The listing builds one solid part. Answer for the finished solid, in the listing's coordinates (mm). A direction names the side the tool comes from. Coordinates: 2 decimals unless noted, no trailing zeros. Loops run counter-clockwise (first coordinate to the right, second up) from the corner with the lowest first, then second, coordinate; pieces in that order, holes last. Notation, with made-up numbers: (82.25, 45.25) - (103.25, 45.25) arc R26 ccw to (103.25, 80.25) - close; hole circle Ø5 at (-13, 5). An arc over 180 degrees is marked (long way). Write each question's results on one line, items separated by ' | '. Start each with the question number.
(1) Given pin 1 Ø2.5 at (x, y) = (0, -5) entering from +Z; pin 2 Ø3 at (x, z) = (0.5, 10) entering from +Y; pin 3 Ø4.5 at (x, y) = (0, 9) entering from -Z, each flat-ended and moving along its own axis, determine where each tip first touches the part or whether it passes through.
(2) Find section D-D on y = -9. Determine the outline of the cut face in (x, z), then the cut area to 3 significant figures.
(3) For faces 4 (the cylindrical face through (-0.07, -3.38, 66.9)), 5 (the flat face through (-0.1, 6.8, 17)), 6 (the flat face through (0, 4, 65)), determine the directions among +Z, -Z, +X, -X, +Y, -Y from which every point of the face is accessible in a straight line to the end or side of a thin tool.
(4) Find section B-B on y = 5.25. Determine the outline of the cut face in (x, z).
(5) Determine the mould class of faces 1 (the conical face through (0.012, -5.281, 14.805)), 2 (the flat face through (0, 6, 47)), 3 (the cylindrical face through (4, 12, 52)) for opening direction Y: released by +Y, released by -Y, zero draft, split by the parting line, or undercut.
(6) Consider line 1 (Z direction, x = 1, y = -9); line 2 (Y direction, x = 0, z = 54.5); line 3 (Z direction, x = 2.25, y = 6.25). Determine where each line is inside the solid, lowest interval first. Write a range as from..to.
(7) Find section A-A on z = 62. Determine the outline of the cut face in (x, y), then the cut area to 3 significant figures.
Autodesk Inventor part; units mm, degrees
ref_plane "YZ Plane" through (0, 0, 0) normal (1, 0, 0) x (0, 1, 0)
ref_plane "XZ Plane" through (0, 0, 0) normal (0, 1, 0) x (-1, 0, 0)
ref_plane "XY Plane" through (0, 0, 0) normal (0, 0, 1) x (1, 0, 0)
sketch "Skizze1" plane through (0, 0, 0) normal (0, 0, 1) x (1, 0, 0)
  line L0 (5, 14) -> (-5, 14)
  line L1 (-5, 14) -> (-5, -14)
  line L2 (-5, -14) -> (5, -14)
  line L3 (5, -14) -> (5, 14)
  line L4 (5, 14) -> (-5, -14) construction
  line L5 (-5, 14) -> (5, -14) construction
  point P0 (0, 0)
  dimension "d0" = 28
  dimension "d1" = 10
extrude "Extrusion1" add sketch "Skizze1" along normal blind 74
sketch "Skizze2" plane through (-5, -14, 0) normal (-1, 0, 0) x (0, 0, 1)
  line L0 (0, 28) -> (74, 28)
  line L1 (0, 28) -> (17, 28)
  line L2 (17, 28) -> (17, 18)
  line L3 (17, 18) -> (0, 18)
  line L4 (0, 18) -> (0, 28)
  line L5 (74, 28) -> (57, 28)
  line L6 (57, 28) -> (57, 18)
  line L7 (57, 18) -> (74, 18)
  line L8 (74, 18) -> (74, 28)
  line L9 (27, 28) -> (47, 28)
  line L10 (47, 28) -> (47, 15)
  line L11 (47, 15) -> (27, 15)
  line L12 (27, 15) -> (27, 28)
  line L13 (0, 0) -> (74, 0)
  point P0 (0, 14)
  dimension "d4" = 15
  dimension "d5" = 20
  dimension "d6" = 40
  dimension "d7" = 10
  dimension "d8" = 18
  dimension "d9" = 18
extrude "Extrusion2" cut sketch "Skizze2" against normal blind 74
sketch "Skizze3" plane through (-5, 4, 57) normal (0, 0, 1) x (1, 0, 0)
  line L0 (10, 10) -> (10, 0)
  line L1 (10, 0) -> (0, 0)
  point P0 (5, -4)
  point P1 (5, 5)
  dimension "d12" = 5
  dimension "d13" = 5
hole "Bohrung1" at (0, 9, 57) direction (0, 0, -1) diameter 4 end through all
fillet "Rundung1" radius 5 4 edges at (-5, 14, 22) (-5, 14, 52) (5, 14, 52) (5, 14, 22)
sketch "Skizze4" plane through (-5, -14, 0) normal (-1, 0, 0) x (0, 0, 1)
  line L0 (0, 18) -> (0, 0)
  line L1 (74, 18) -> (74, 0)
  line L2 (74, 18) -> (57, 18)
  point P0 (0, 14)
  point P1 (12, 5)
  point P2 (62, 5)
  dimension "d22" = 50
  dimension "d23" = 12
  dimension "d24" = 12
  dimension "d25" = 13
hole "Bohrung2" at (-5, -9, 12) at (-5, -9, 62) direction (1, 0, 0) diameter 3 end through all
sketch "Skizze5" plane through (0, 0, 74) normal (0, 0, 1) x (1, 0, 0)
  line L0 (-5, -14) -> (5, -14)
  line L1 (-5, 4) -> (-5, -14)
  point P0 (0, 0)
  point P1 (0, -5)
  dimension "d33" = 9
  dimension "d34" = 5
hole "Bohrung3" at (0, -5, 74) direction (0, 0, -1) diameter 3.242 depth 14 tip angle 118
sketch "Skizze6" plane through (0, 0, 0) normal (0, 0, -1) x (-1, 0, 0)
  line L0 (5, 4) -> (5, -14)
  line L1 (5, -14) -> (-5, -14)
  point P0 (0, 0)
  point P1 (0, -5)
  dimension "d42" = 5
  dimension "d43" = 9
hole "Bohrung4" at (0, -5, 0) direction (0, 0, 1) diameter 3.242 depth 14 tip angle 118
properties part number "ABI_Lagerbock"
Values:
1) pin 1: stops at z = 59.78 | pin 2: stops at y = 4 | pin 3: stops at z = 17
2) outline: (-5, 0) - (5, 0) - (5, 10.5) - (-5, 10.5) - close; (-5, 13.5) - (5, 13.5) - (5, 60.5) - (-5, 60.5) - close; (-5, 63.5) - (5, 63.5) - (5, 74) - (-5, 74) - close | area: 680 mm²
3) face 4: +Z | face 5: -Z, +X, -X, +Y | face 6: +Z, +X, -X, +Y
4) outline: (-5, 17) - (5, 17) - (5, 27) - (-5, 27) - close; (-5, 47) - (5, 47) - (5, 57) - (-5, 57) - close
5) face 1: undercut | face 2: zero draft | face 3: released by +Y
6) line 1: z = 0..10.5, 13.5..60.5, 63.5..74 | line 2: y = -14..7, 11..14 | line 3: z = 17..27, 47..57
7) outline: (-5, -14) - (5, -14) - (5, -10.5) - (-5, -10.5) - close; (-5, -7.5) - (5, -7.5) - (5, 4) - (-5, 4) - close; hole circle Ø3.24 at (0, -5) | area: 142 mm²
